CAD build for the part. Positions are in the model's coordinates, mm. A direction names the side the tool comes from. Coordinates: 2 decimals unless noted, no trailing zeros. Write each loop counter-clockwise with the first axis right and the second up, starting at its lowest first coordinate (ties: lowest second). Pieces come first, ordered by that corner, then holes. Notation, with made-up numbers: (64.25, 24) - (88.25, 24) arc R20 cw to (88.25, 33) - close; hole circle Ø4 at (-35.5, 20.5). An arc over 180 degrees is marked (long way). Answer in a Markdown table with one row per item. Add a question column.
Q1. Drill centre lines: line 1 along Y through (x, z) = (17, 47); line 2 along Z through (x, y) = (9.5, -13); line 3 along Y through (x, z) = (23, 37.5). Where is each one in solid material? Low to high. Write a range as from..to.
Q2. Band-saw the part on A-A (x = 22). List the corners of the cut face in (y, z), and give its area (3 significant figures).
Q3. 3-axis set-ups, long thin cutter, end or side, ignore diameter. For faces 1 (the flat face through (0, 9.534, 48)), 2 (the flat face through (-13, -11.097, 48)), 3 (the flat face through (25.4, 0, -2)): which of +Z, -Z, +X, -X, +Y, -Y reach the whole face in a straight line?
Q4. Pin check, flat tips, straight feed: pin 1 (6 mm diameter, centred on y = 15, z = 39.5, fed in from +X); pin 2 (2.5 mm diameter, centred on x = 8.5, z = 49, fed in from -Y); pin 3 (4.5 mm diameter, centred on x = 6, z = 48, fed in from +Y). Stop position of each tip, or through.
```python
from build123d import *

# Parameters (mm, degrees)
F1_DEPTH = 25.4
F2_DEPTH = 25.4


with BuildPart() as f1:
    # F0 (on Right) → F1 (new body)
    with BuildSketch(Plane.YZ):
        Polygon((9.533734, 52.669968), (0, 52.669968), (-11.09664, 52.669968), (-11.09664, 43.605104), (9.533734, 43.605104), align=None)
        Polygon((20.161506, 32.664757), (9.533734, 43.605104), (-11.09664, 43.605104), (-18.911175, 32.664757), (-18.911175, -58.296442), (0, -58.296442), (20.161506, -58.296442), align=None)
    extrude(amount=F1_DEPTH)

    # F1_face (on face) → F2 (join)
    with BuildSketch(Plane(origin=(0, 0.509843, -5.968022), x_dir=(0, 1, 0), z_dir=(-1, 0, 0))):
        Polygon((-11.606484, -58.63799), (9.023891, -58.63799), (9.023891, -49.573126), (19.651662, -38.632779), (19.651662, 52.32842), (-19.421019, 52.32842), (-19.421019, -38.632779), (-11.606484, -49.573126), align=None)
    extrude(amount=F2_DEPTH)


solid = f1.part
```
Checked values:
| question | item | result |
|---|---|---|
| 1 | line 1 | y = -11.1..9.53 |
| 1 | line 2 | z = -58.3..40.94 |
| 1 | line 3 | y = -15.46..15.46 |
| 2 | outline | (-18.91, -58.3) - (20.16, -58.3) - (20.16, 32.66) - (9.53, 43.61) - (9.53, 52.67) - (-11.1, 52.67) - (-11.1, 43.61) - (-18.91, 32.66) - close |
| 2 | area | 4,070 mm² |
| 3 | face 1 | +Z, +X, -X, +Y |
| 3 | face 2 | +Z, +X, -X, -Y |
| 3 | face 3 | +Z, -Z, +X, +Y, -Y |
| 4 | pin 1 | stops at x = 25.4 |
| 4 | pin 2 | stops at y = -11.1 |
| 4 | pin 3 | stops at y = 9.53 |
